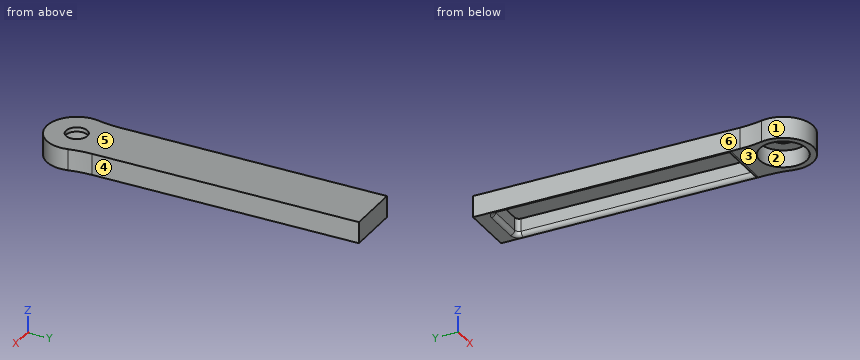
```python
from build123d import *

# Parameters (mm, degrees)
SKETCH2_R           = 11
BOSS_EXTRUDE1_DEPTH = 10
BOSS_EXTRUDE3_START = 2
SKETCH6_R           = 11
SKETCH6_R_2         = 5
BOSS_EXTRUDE3_DEPTH = 2
SKETCH11_W          = 21
SKETCH11_H          = 110
CUT_EXTRUDE1_DEPTH  = 8
FILLET2_R           = 50
FILLET3_R           = 2


with BuildPart() as part:
    # Sketch2 → Boss-Extrude1 (new body)
    with BuildSketch(Plane.XY):
        with BuildLine():
            Line((12.5, 138.478281378), (-12.5, 138.478281378))
            Line((-12.5, 138.478281378), (-12.5, 6.304760106))
            ThreePointArc((-12.5, 6.304760106), (0, -14), (12.5, 6.304760106))
            Line((12.5, 6.304760106), (12.5, 138.478281378))
        make_face()
        Circle(SKETCH2_R, mode=Mode.SUBTRACT)
    extrude(amount=BOSS_EXTRUDE1_DEPTH)

    # Sketch6 → Boss-Extrude3 (add)
    with BuildSketch(Plane(origin=(0, 0, 10), x_dir=(-1, 0, 0), z_dir=(0, 0, -1)).offset(BOSS_EXTRUDE3_START)):
        Circle(SKETCH6_R)
        Circle(SKETCH6_R_2, mode=Mode.SUBTRACT)
    extrude(amount=-BOSS_EXTRUDE3_DEPTH)

    # Sketch11 → Cut-Extrude1 (cut)
    with BuildSketch(Plane(origin=(0, 0, 0), x_dir=(-1, 0, 0), z_dir=(0, 0, -1))):
        with Locations((0, 75)):
            Rectangle(SKETCH11_W, SKETCH11_H)
    extrude(amount=-CUT_EXTRUDE1_DEPTH, mode=Mode.SUBTRACT)

    # Fillet2
    fillet2_edges = [part.edges().sort_by_distance(p)[0] for p in [
        (12.5, 6.304760106, 5),
        (-12.5, 6.304760106, 5),
    ]]
    fillet(fillet2_edges, radius=FILLET2_R)

    # Fillet3
    fillet3_edges = [part.edges().sort_by_distance(p)[0] for p in [
        (10.5, 75, 0),
        (0, 20, 0),
        (-10.5, 75, 0),
        (0, 130, 0),
        (-10.5, 130, 4),
        (10.5, 130, 4),
    ]]
    fillet(fillet3_edges, radius=FILLET3_R - 0.0001)  # a hair under: the kernel refuses the full size


solid = part.part
```
Part model, mm, in its own coordinate system. Face numbers are marked on the shaded views. A direction names the side the tool comes from. Coordinates: 2 decimals unless noted, no trailing zeros. Write each loop counter-clockwise with the first axis right and the second up, starting at its lowest first coordinate (ties: lowest second). Pieces come first, ordered by that corner, then holes.
Item 1: Slice it at A-A (y = 0). Write the cut outline in (x, z).
Item 2: Probe line 1 (Y direction, x = 0, z = 2.75); line 2 (X direction, y = 0, z = 5.75); line 3 (Y direction, x = -8.25, z = 2). List the from-to ranges inside material, lowest first.
Item 3: Which spindle directions (+Z, -Z, +X, -X, +Y, -Y) get a long thin tool onto all of the face, cutting with end or side? Do the marked faces 4, 5 and 6. Say none if no direction does.
Item 4: Slice it at B-B (x = 0). Write the cut outline in (y, z), and give its area (3 significant figures).
Item 5: Pin check, flat tips, straight feed: pin 1 (1.8 mm diameter, centred on y = 69.5, z = 4, fed in from +X); pin 2 (4 mm diameter, centred on y = 46, z = 1.5, fed in from -X); pin 3 (11.5 mm diameter, centred on x = 0, y = 0, fed in from -Z). Stop position of each tip, or through.
Item 6: Slice it at C-C (z = 5.5). Write the cut outline in (x, y).
Item 7: Mould opens along X. For the marked faces 1, 2 and 3 say: released by +X, released by -X, zero draft, split by the parting line, or undercut.
Results found:
1. outline: (-14, 0) - (-11, 0) - (-11, 8) - (-5, 8) - (-5, 10) - (-14, 10) - close; (5, 8) - (11, 8) - (11, 0) - (14, 0) - (14, 10) - (5, 10) - close
2. line 1: y = -14 to -11, 11 to 20, 130 to 138.48
2. line 2: x = -14 to -11, 11 to 14
2. line 3: y = -11.31 to -7.28, 7.28 to 20, 130 to 138.48
3. face 4: +Z, -Z, +X, +Y
3. face 5: +Z, +X, -X, +Y, -Y
3. face 6: +Z, -Z, -X, +Y
4. outline: (-14, 0) - (-11, 0) - (-11, 8) - (-5, 8) - (-5, 10) - (-14, 10) - close; (5, 8) - (11, 8) - (11, 0) - (18, 0) arc R2 ccw to (20, 2) - (20, 8) - (130, 8) - (130, 2) arc R2 ccw to (132, 0) - (138.48, 0) - (138.48, 10) - (5, 10) - close
4. area: 447 mm2
5. pin 1: stops at x = 12.5
5. pin 2: stops at x = -12.5
5. pin 3: stops at z = 8
6. outline: (-13.67, 3.01) arc R14 ccw (long way) to (13.67, 3.01) arc R50 cw to (12.5, 13.77) - (12.5, 138.48) - (-12.5, 138.48) - (-12.5, 13.77) arc R50 cw to start; hole circle Ø22 at (0, 0); hole (-10.5, 20) - (10.5, 20) - (10.5, 128) arc R2 ccw to (8.5, 130) - (-8.5, 130) arc R2 ccw to (-10.5, 128) - close
7. face 1: split by the parting line
7. face 2: undercut
7. face 3: zero draft
